from build123d import *

# Parameters (mm, degrees)
SKETCH024_R           = 14
SKETCH024_R_2         = 2.5
PAD006_DEPTH          = 10
PAD007_DEPTH          = 4
SKETCH026_R           = 1.5
POCKET011_DEPTH       = 5
POLARPATTERN001_COUNT = 3
PAD008_DEPTH          = 5
POLARPATTERN002_COUNT = 3
SKETCH031_W           = 6
SKETCH031_H           = 7
POCKET013_DEPTH       = 155.736206
POLARPATTERN005_COUNT = 3
CHAMFER_SIZE          = 5
SKETCH048_R           = 2
POCKET020_DEPTH       = 5
POLARPATTERN009_COUNT = 3
POCKET027_DEPTH       = 4
POLARPATTERN010_COUNT = 3
SKETCH060_R           = 12
POCKET028_DEPTH       = 5
SKETCH116_R           = 5
POCKET076_DEPTH       = 3


with BuildPart() as part:
    # Sketch024 → Pad006 (new body)
    with BuildSketch(Plane.XY):
        Circle(SKETCH024_R)
        Circle(SKETCH024_R_2, mode=Mode.SUBTRACT)
    extrude(amount=-PAD006_DEPTH)

    # Sketch025 → Pad007 (join)
    with BuildSketch(Plane.XZ.offset(2.1)):
        with BuildLine():
            ThreePointArc((-21.82274, 8.677566), (-19.999991, -2.452603), (-10.028464, -7.722494))
            ThreePointArc((-10.028464, -7.722494), (-5.929578, -3.823887), (-9.828184, 0.274999))
            ThreePointArc((-14.17726, 6.322434), (-13.505131, 2.218243), (-9.828184, 0.274999))
            ThreePointArc((-14.17726, 6.322434), (-16.822434, 11.32274), (-21.82274, 8.677566))
        make_face()
    extrude(amount=PAD007_DEPTH)

    # Sketch026 (on Face5 of Pad007) → Pocket011 (cut)
    with BuildSketch(Plane.XZ.offset(6.1)):
        with Locations((-17.973509, 7.445274)):
            Circle(SKETCH026_R)
    extrude(amount=-POCKET011_DEPTH, mode=Mode.SUBTRACT)

    # Mirrored003: part across XZ


with BuildPart() as part_1:
    add(part.part)
    add(part.part.mirror(Plane.XZ))

    # PolarPattern001: part ×3 about axis
    polarpattern001_axis = Axis((0, 0, 0), (0, 0, 1))


with BuildPart() as part_2:
    add(part_1.part)
    for i in range(1, POLARPATTERN001_COUNT):
        add(part_1.part.rotate(polarpattern001_axis, i * 360 / POLARPATTERN001_COUNT))

    # Sketch027 (on Face1 of PolarPattern001) → Pad008 (join)
    with BuildSketch(Plane.XY):
        with BuildLine():
            ThreePointArc((-0.000709, 22), (-11.000814, 19.052089), (-19.053145, 10.998985))
            Line((-19.053145, 10.998985), (-11.258916, 6.498985))
            ThreePointArc((-0.000709, 13), (-6.500814, 11.25786), (-11.258916, 6.498985))
            Line((-0.000709, 22), (-0.000709, 13))
        make_face()
    pad008 = extrude(amount=PAD008_DEPTH)

    # PolarPattern002: Pad008 ×3 about axis
    polarpattern002_axis = Axis((0, 0, 0), (0, 0, 1))
    for i in range(1, POLARPATTERN002_COUNT):
        add(pad008.rotate(polarpattern002_axis, i * 360 / POLARPATTERN002_COUNT))

    # Sketch031 → Pocket013 (cut, through all)
    with BuildSketch(Plane.YZ):
        with Locations((0, 18.5)):
            Rectangle(SKETCH031_W, SKETCH031_H)
    pocket013 = extrude(amount=-POCKET013_DEPTH, mode=Mode.SUBTRACT)

    # PolarPattern005: Pocket013 ×3 about axis
    polarpattern005_axis = Axis((0, 0, 0), (0, 0, 1))
    for i in range(1, POLARPATTERN005_COUNT):
        add(pocket013.rotate(polarpattern005_axis, i * 360 / POLARPATTERN005_COUNT), mode=Mode.SUBTRACT)

    # Chamfer
    chamfer_edges = [part_2.edges().sort_by_distance(p)[0] for p in [
        (-3.623809, 13.52287, 0),
        (-9.899909, 9.899081, 0),
        (-9.899244, -9.899746, 0),
        (-3.622901, -13.523113, 0),
        (13.52281, 3.624033, 0),
        (13.523053, -3.623124, 0),
    ]]
    chamfer(chamfer_edges, length=CHAMFER_SIZE)

    # Sketch048 (on Face37 of Chamfer) → Pocket020 (cut)
    with BuildSketch(Plane.XY.offset(5)):
        with Locations((15, 0)):
            Circle(SKETCH048_R)
    pocket020 = extrude(amount=-POCKET020_DEPTH, mode=Mode.SUBTRACT)

    # PolarPattern009: Pocket020 ×3 about axis
    polarpattern009_axis = Axis((0, 0, 5), (0, 0, 1))
    for i in range(1, POLARPATTERN009_COUNT):
        add(pocket020.rotate(polarpattern009_axis, i * 360 / POLARPATTERN009_COUNT), mode=Mode.SUBTRACT)

    # Sketch059 (on Face39 of PolarPattern009) → Pocket027 (cut)
    with BuildSketch(Plane(origin=(0, -2.1, 0), x_dir=(-1, 0, 0), z_dir=(0, 1, 0))):
        with BuildLine():
            ThreePointArc((23.463233, -4.296317), (20.141453, 20.322409), (9, -1.880832))
            Line((9, -1.880832), (9, -14.311207))
            Line((9, -14.311207), (23.463233, -14.311207))
            Line((23.463233, -14.311207), (23.463233, -4.296317))
        make_face()
    pocket027 = extrude(amount=POCKET027_DEPTH, mode=Mode.SUBTRACT)

    # PolarPattern010: Pocket027 ×3 about axis
    polarpattern010_axis = Axis((0, 0, 0), (0, 0, 1))
    for i in range(1, POLARPATTERN010_COUNT):
        add(pocket027.rotate(polarpattern010_axis, i * 360 / POLARPATTERN010_COUNT), mode=Mode.SUBTRACT)

    # Sketch060 (on Face7 of PolarPattern010) → Pocket028 (cut)
    with BuildSketch(Plane.XY.offset(1)):
        Circle(SKETCH060_R)
    extrude(amount=-POCKET028_DEPTH, mode=Mode.SUBTRACT)

    # Sketch116 (on Face24 of Pocket028) → Pocket076 (cut)
    with BuildSketch(Plane.XY.offset(-4)):
        Circle(SKETCH116_R)
    extrude(amount=-POCKET076_DEPTH, mode=Mode.SUBTRACT)


with BuildPart() as part_3:
    # Body004 placement: moved
    add(part_2.part.moved(Location((0, 0, -28))))


solid = part_3.part
Read the model definition and answer for the solid it produces. Units are mm, in the model's axes. A direction names the side the tool comes from. Give positions to 0.01 mm unless a question says otherwise; leave off trailing zeros. Loops run counter-clockwise (first coordinate to the right, second up) from the corner with the lowest first, then second, coordinate; pieces in that order, holes last. Notation, with made-up numbers: (31, -14.5) -> (69, -14.5) arc R21 ccw to (69, 24.5) -> close; hole circle Ø7 at (15, -38). An arc over 180 degrees is marked (long way). Answer as CSV lines item,"result".
Item 1: Find section B-B on x = -18. Give the vertices of the cut face in (y, z), plus the area to 3 significant figures.
Returned:
outline,"(-12.65, -28) -> (-10.39, -28) -> (-10.39, -23) -> (-12.65, -23) -> close; (-6.1, -32.64) -> (-2.1, -32.64) -> (-2.1, -22.05) -> (-6.1, -22.05) -> close; (-6.1, -19.05) -> (-2.1, -19.05) -> (-2.1, -16.5) -> (-6.1, -16.5) -> close; (2.1, -32.64) -> (6.1, -32.64) -> (6.1, -22.05) -> (2.1, -22.05) -> close; (2.1, -19.05) -> (6.1, -19.05) -> (6.1, -16.5) -> (2.1, -16.5) -> close; (10.39, -28) -> (12.65, -28) -> (12.65, -23) -> (10.39, -23) -> close"
area,"128 mm²"
Item 2: For faces 1 (the face through (7.617, 9.392, -34.041)), 2 (the face through (12.3, 0.1, -28)), 3 (the face through (-13.68, -4.07, -25.52)), determine the directions among +Z, -Z, +X, -X, +Y, -Y from which every point of the face is accessible in a straight line to the end or side of a thin tool.
Returned:
face 1,"+Z, -Z"
face 2,"+Z"
face 3,"none"
Item 3: Consider line 1 (Y direction, x = 0, z = -37.35); line 2 (Y direction, x = 15, z = -26.4); line 3 (X direction, y = -16.5, z = -23.75). Determine where each line is inside the solid, lowest interval first. Write a range as [from, to].
Returned:
line 1,"y = [-14, -2.5], [2.5, 14]"
line 2,"y = [-16.67, -13.78], [-8.66, -2], [2, 8.66], [13.78, 16.67]"
line 3,"x = [-14.55, 0], [2.48, 7.1], [11.95, 16.15]"
Item 4: Each of these flat-tipped pins is pushed along its axis until it touches: pin 1 (4 mm diameter, centred on x = -12, y = 18.5, fed in from -Z); pin 2 (12.5 mm diameter, centred on x = -8.5, y = 17.5, fed in from +Z); pin 3 (0.6 mm diameter, centred on x = 4.5, y = -12, fed in from +Z). Where does it stop, or does it pass through?
Returned:
pin 1,"stops at z = -28"
pin 2,"stops at z = -23"
pin 3,"stops at z = -26.43"
Item 5: Find section A-A on z = -36.5. Give the vertices of the cut face in (x, y).
Returned:
outline,"(-13.87, 1.9) -> (-9, 1.9) -> (-9, -2.1) -> (-13.84, -2.1) arc R14 ccw to (5.29, -12.96) -> (2.85, -8.74) -> (6.32, -6.74) -> (8.74, -10.94) arc R14 ccw to (8.58, 11.06) -> (6.15, 6.84) -> (2.68, 8.84) -> (5.1, 13.04) arc R14 ccw to start; hole circle Ø5 at (0, 0)"
Item 6: Determine the mould class of faces 4 (the face through (-15.21, -8.782, -26.959)), 5 (the face through (-6.3, 10.4, -28)), 6 (the face through (-8, -16, -23)) for opening direction X: +X half, -X half, draft (parallel to the pull), parting line (faces both ways), or undercut.
Returned:
face 4,"-X half"
face 5,"undercut"
face 6,"draft"
